Input: part model. Units: mm. Frame: model coordinates. A direction names the side the tool comes from. Coordinates: 2 decimals unless noted, no trailing zeros. Loops run counter-clockwise (first coordinate to the right, second up) from the corner with the lowest first, then second, coordinate; pieces in that order, holes last.
Item 1: Ray query, line 1 along Z through (x, y) = (11.5, -1); line 2 along Y through (x, z) = (0, -81); line 3 along X through (y, z) = (-4, -43). Return the intervals inside material, ascending.
Item 2: Pull-direction query (X, two-part tool) for faces 1 (the cylindrical face through (-10.395, 0.181, -66.008)), 2 (the flat face through (0, -2, 0)), 3 (the flat face through (5.72, -17.53, -9.39)); classes: released by +X, released by -X, zero draft, split by the parting line, or undercut.
Item 3: Section A-A on z = -14. Return loops of the section in (x, y), and give its area (3 significant figures).
Item 4: Section D-D on z = -47.5. Return loops of the section in (x, y), and give its area (3 significant figures).
Item 5: Contact query for flat-ended pins moving along their axis: P1, Ø6, axis at y = -8, z = -9.5, coming from the -X side; P2, Ø6, axis at x = 1, z = -66, coming from the +Y side; P3, Ø12, axis at x = -2.5, z = -86.5, coming from the -Y side. Output: stop coordinate, or through.
Item 6: Reachability of faces 4 (the flat face through (0, -7.302, -66)), 5 (the flat face through (-14.924, -11, -9)), 6 (the flat face through (0, 7.434, -66)) from +Z, -Z, +X, -X, +Y, -Y: full face, straight path, thin tool, end or side. Return the list, or none.
Item 7: Section B-B on x = 5.5. Return loops of the section in (y, z), and give its area (3 significant figures).
Item 8: Section C-C on y = 19. Return loops of the section in (x, z), and give its area (3 significant figures).
```python
from build123d import *

# Parameters (mm, degrees)
BOSS_EXTRUDE1_DEPTH = 114.3
BOSS_EXTRUDE2_DEPTH = 19.05


with BuildPart() as part:
    # Sketch1 → Boss-Extrude1 (new body)
    with BuildSketch(Plane.XY):
        with BuildLine():
            Line((-7.341079337, -7.302244278), (7.377825429, -7.302244278))
            ThreePointArc((7.377825429, -7.302244278), (10.432373046, 0.065920801), (7.377825429, 7.434085879))
            Line((7.377825429, 7.434085879), (-7.341079337, 7.434085879))
            ThreePointArc((-7.341079337, 7.434085879), (-10.395626954, 0.065920801), (-7.341079337, -7.302244278))
        make_face()
    extrude(amount=-BOSS_EXTRUDE1_DEPTH)

    # Sketch2 → Boss-Extrude2 (add)
    with BuildSketch(Plane.XY):
        with BuildLine():
            Line((-11.594830289, -19.452818555), (0, -15.661809823))
            Line((0, -15.661809823), (11.594830289, -19.452818555))
            ThreePointArc((11.594830289, -19.452818555), (13.875262434, -19.094861422), (14.924180561, -17.038584484))
            Line((14.924180561, -17.038584484), (14.924180561, -4.642008184))
            Line((14.924180561, -4.642008184), (22.032123103, 4.98159964))
            ThreePointArc((22.032123103, 4.98159964), (22.40396274, 7.277739061), (20.750529859, 8.913795499))
            Line((20.750529859, 8.913795499), (9.373214352, 12.489409744))
            Line((9.373214352, 12.489409744), (2.054903166, 22.56220095))
            ThreePointArc((2.054903166, 22.56220095), (0, 23.609226409), (-2.054903166, 22.56220095))
            Line((-2.054903166, 22.56220095), (-9.373214352, 12.489409744))
            Line((-9.373214352, 12.489409744), (-20.750529859, 8.913795499))
            ThreePointArc((-20.750529859, 8.913795499), (-22.40396274, 7.277739061), (-22.032123103, 4.98159964))
            Line((-22.032123103, 4.98159964), (-14.924180561, -4.642008184))
            Line((-14.924180561, -4.642008184), (-14.924180561, -17.038584484))
            ThreePointArc((-14.924180561, -17.038584484), (-13.875262434, -19.094861422), (-11.594830289, -19.452818555))
        make_face()
    extrude(amount=-BOSS_EXTRUDE2_DEPTH)


solid = part.part
```
Results found:
1. line 1: z = -19.05 to 0
1. line 2: y = -7.3 to 7.43
1. line 3: x = -9.57 to 9.61
2. face 1: released by -X
2. face 2: zero draft
2. face 3: undercut
3. outline: (-22.03, 4.98) - (-14.92, -4.64) - (-14.92, -17.04) arc R2.54 ccw to (-11.59, -19.45) - (0, -15.66) - (11.59, -19.45) arc R2.54 ccw to (14.92, -17.04) - (14.92, -4.64) - (22.03, 4.98) arc R2.54 ccw to (20.75, 8.91) - (9.37, 12.49) - (2.05, 22.56) arc R2.54 ccw to (-2.05, 22.56) - (-9.37, 12.49) - (-20.75, 8.91) arc R2.54 ccw to start
3. area: 1,150 mm2
4. outline: (-7.34, -7.3) - (7.38, -7.3) arc R10.41 ccw to (7.38, 7.43) - (-7.34, 7.43) arc R10.41 ccw to start
4. area: 279 mm2
5. P1: stops at x = -14.92
5. P2: stops at y = 7.43
5. P3: stops at y = -7.3
6. face 4: -Z, +X, -X, -Y
6. face 5: +Z, -Z, -X, -Y
6. face 6: -Z, +X, -X, +Y
7. outline: (-17.46, -19.05) - (-7.3, -19.05) - (-7.3, -114.3) - (7.43, -114.3) - (7.43, -19.05) - (17.82, -19.05) - (17.82, 0) - (-17.46, 0) - close
7. area: 2,080 mm2
8. outline: (-4.64, -19.05) - (4.64, -19.05) - (4.64, 0) - (-4.64, 0) - close
8. area: 177 mm2
